Design review of the part built by this model. Coordinates are the model's own, in mm. Face numbers are marked on the shaded views. A direction names the side the tool comes from. Coordinates: 2 decimals unless noted, no trailing zeros. Order: outer loops, then holes, each group sorted by start corner. A loop starts at its lowest first (then second) coordinate and runs counter-clockwise, first axis right, second up. Notation, with made-up numbers: M 9.5,87.25 L 32.5,87.25 A8 cw 32.5,93.25 Z; hole C -23.75,-30 d11. An arc over 180 degrees is marked long. Use CSV: the item, a comma, the result in double quotes.
```python
from build123d import *

# Parameters (mm, degrees)
SKETCH1_W           = 76
SKETCH1_H           = 56
BOSS_EXTRUDE1_DEPTH = 3
SKETCH2_W           = 76
SKETCH2_H           = 56
SKETCH2_W_2         = 70
SKETCH2_H_2         = 50
BOSS_EXTRUDE2_DEPTH = 28
CUT_EXTRUDE1_REACH  = 88.724
SKETCH3_W           = 25
SKETCH3_H           = 10
BOSS_EXTRUDE3_START = 31
SKETCH4_W           = 70
SKETCH4_H           = 50
SKETCH4_W_2         = 64
SKETCH4_H_2         = 49.98
BOSS_EXTRUDE3_DEPTH = 8
SKETCH5_R           = 0.85
CUT_EXTRUDE2_DEPTH  = 5


with BuildPart() as part:
    # Sketch1 → Boss-Extrude1 (new body)
    with BuildSketch(Plane(origin=(0, 0, 0), x_dir=(1, 0, 0), z_dir=(0, 1, 0))):
        Rectangle(SKETCH1_W, SKETCH1_H)
    extrude(amount=BOSS_EXTRUDE1_DEPTH)

    # Sketch2 → Boss-Extrude2 (add)
    with BuildSketch(Plane(origin=(0, 3, 0), x_dir=(1, 0, 0), z_dir=(0, 1, 0))):
        Rectangle(SKETCH2_W, SKETCH2_H)
        Rectangle(SKETCH2_W_2, SKETCH2_H_2, mode=Mode.SUBTRACT)
    extrude(amount=BOSS_EXTRUDE2_DEPTH)

    # Sketch3 → Cut-Extrude1 (cut, up to next)
    with BuildSketch(Plane.ZY.offset(38), mode=Mode.PRIVATE) as cut_extrude1_sk1:
        with Locations((0, 8)):
            Rectangle(SKETCH3_W, SKETCH3_H)
    cut_extrude1_tool1 = extrude(cut_extrude1_sk1.sketch, amount=-CUT_EXTRUDE1_REACH, mode=Mode.PRIVATE) & part.part
    add(cut_extrude1_tool1.solids().sort_by_distance((-38, 8, 0))[0], mode=Mode.SUBTRACT)

    # Sketch4 → Boss-Extrude3 (add)
    with BuildSketch(Plane(origin=(0, 0, 0), x_dir=(1, 0, 0), z_dir=(0, 1, 0)).offset(BOSS_EXTRUDE3_START)):
        Rectangle(SKETCH4_W, SKETCH4_H)
        Rectangle(SKETCH4_W_2, SKETCH4_H_2, mode=Mode.SUBTRACT)
    extrude(amount=-BOSS_EXTRUDE3_DEPTH)

    # Sketch5 → Cut-Extrude2 (cut)
    with BuildSketch(Plane(origin=(0, 31, 0), x_dir=(1, 0, 0), z_dir=(0, 1, 0))):
        with Locations(Location((-35, 0, 0), (0, 0, 270))):
            Circle(SKETCH5_R)
        with Locations(Location((35, 0, 0), (0, 0, 90))):
            Circle(SKETCH5_R)
    extrude(amount=-CUT_EXTRUDE2_DEPTH, mode=Mode.SUBTRACT)


solid = part.part
```
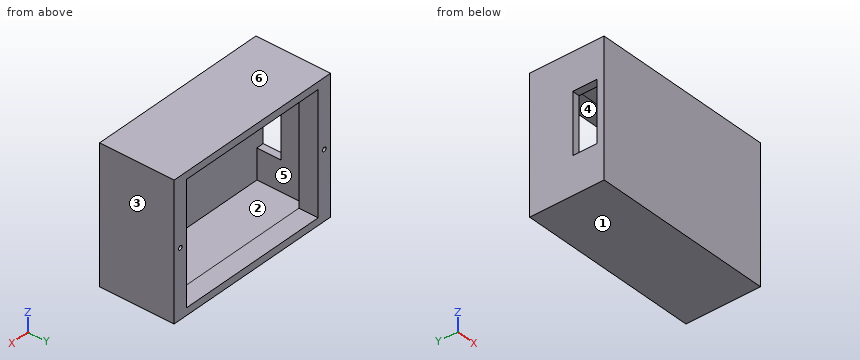
(1) The part is to be moulded in two halves that separate along X. For the marked faces 1, 2 and 3, say which applies: pulls with the +X half, pulls with the -X half, needs draft (parallel to the pull), parting line crosses it, or undercut.
The answers:
face 1,"needs draft"
face 2,"undercut"
face 3,"pulls with the +X half"
(2) For the marked faces 4, 5 and 6, list the 3-axis set-ups (+Z, -Z, +X, -X, +Y, -Y) from which the entire face can be reached by the end or side of a thin tool; tool diameter is ignored.
The answers:
face 4,"+Y"
face 5,"none"
face 6,"+Z, +X, -X, +Y, -Y"
(3) Add section B-B on y = 19. State the section outline as (x, z) points, and give its area (3 significant figures).
The answers:
outline,"M -38,-28 L 38,-28 L 38,28 L -38,28 Z; hole M -35,-25 L 35,-25 L 35,25 L -35,25 Z"
area,"756 mm2"
(4) Add section A-A on z = 0. State the section outline as (x, y) points, and give its area (3 significant figures).
The answers:
outline,"M -38,0 L 38,0 L 38,31 L 35.85,31 L 35.85,26 L 34.15,26 L 34.15,31 L 32,31 L 32,23 L 35,23 L 35,3 L -38,3 Z; M -38,13 L -35,13 L -35,23 L -32,23 L -32,31 L -34.15,31 L -34.15,26 L -35.85,26 L -35.85,31 L -38,31 Z"
area,"397 mm2"
(5) Add section C-C on y = 10.5. State the section outline as (x, z) points.
The answers:
outline,"M -38,-28 L 38,-28 L 38,28 L -38,28 L -38,12.5 L -35,12.5 L -35,25 L 35,25 L 35,-25 L -35,-25 L -35,-12.5 L -38,-12.5 Z"
(6) Wall thickness on probe 1 along X at (y, z) = (27.3, 0); probe 2 along Z at (x, y) = (-34, 5.5); probe 3 along X at (y, z) = (6, -14): over which ranges is each line inside the solid? List them lowest first.
The answers:
probe 1,"x = -38 to -35.85, -34.15 to -32, 32 to 34.15, 35.85 to 38"
probe 2,"z = -28 to -25, 25 to 28"
probe 3,"x = -38 to -35, 35 to 38"
(7) Clearance check with flat-ended pins moving along their axes: P1, Ø2, axis at x = -35, z = 0, coming from the -Y side; P2, Ø6, axis at x = -20, z = -1.5, coming from the +Y side. State where each tip first meets the part, or that it passes through.
The answers:
P1,"stops at y = 0"
P2,"stops at y = 3"
(8) Add section D-D on z = -21. State the section outline as (x, y) points, and give its area (3 significant figures).
The answers:
outline,"M -38,0 L 38,0 L 38,31 L 32,31 L 32,23 L 35,23 L 35,3 L -35,3 L -35,23 L -32,23 L -32,31 L -38,31 Z"
area,"444 mm2"
